Verification items for the finished model (mm, model axes). Face numbers are marked on the shaded views. A direction names the side the tool comes from. Round coordinates to 2 decimals unless told otherwise and drop trailing zeros. Order: outer loops, then holes, each group sorted by start corner. A loop starts at its lowest first (then second) coordinate and runs counter-clockwise, first axis right, second up. Notation, with made-up numbers: (-34, 68.25) -> (-30, 68.25) arc R18 ccw to (-30, 84.25) -> close; hole circle Ø4 at (-12.5, -2). An arc over 180 degrees is marked (long way). Put each result on its own line as item: value.
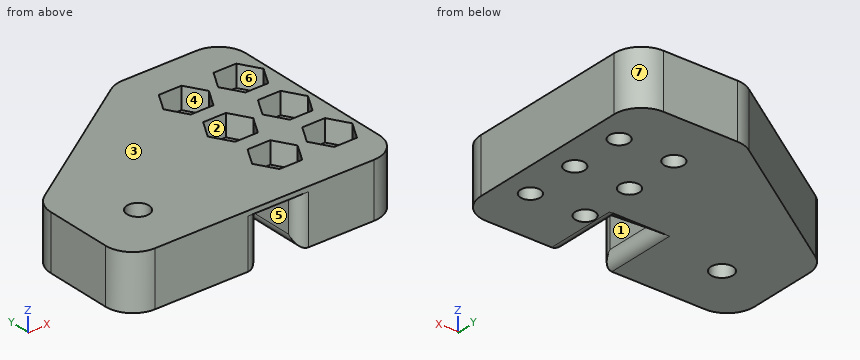
from build123d import *

# Parameters (mm, degrees)
SKETCH1_R           = 2.286
SKETCH1_R_2         = 2.54
BOSS_EXTRUDE1_DEPTH = 12.7
FILLET1_R           = 6.35
CUT_EXTRUDE1_DEPTH  = 8.89
FILLET2_R           = 2.54
CUT_EXTRUDE2_DEPTH  = 5.08


with BuildPart() as part:
    # Sketch1 → Boss-Extrude1 (new body)
    with BuildSketch(Plane.XY):
        Polygon((-6.35, 38.1), (-44.45, 12.7), (-44.45, -12.7), (-6.35, -12.7), (19.05, -12.7), (19.05, 38.1), align=None)
        Circle(SKETCH1_R, mode=Mode.SUBTRACT)
        with Locations((-31.75, 0)):
            Circle(SKETCH1_R_2, mode=Mode.SUBTRACT)
        with Locations((12.7, 0)):
            Circle(SKETCH1_R, mode=Mode.SUBTRACT)
        with Locations((12.7, 12.7)):
            Circle(SKETCH1_R, mode=Mode.SUBTRACT)
        with Locations((12.7, 25.4)):
            Circle(SKETCH1_R, mode=Mode.SUBTRACT)
        with Locations((0, 12.7)):
            Circle(SKETCH1_R, mode=Mode.SUBTRACT)
        with Locations((0, 25.4)):
            Circle(SKETCH1_R, mode=Mode.SUBTRACT)
    extrude(amount=BOSS_EXTRUDE1_DEPTH)

    # Fillet1
    fillet1_edges = [part.edges().sort_by_distance(p)[0] for p in [
        (-44.45, -12.7, 6.35),
        (-44.45, 12.7, 6.35),
        (-6.35, 38.1, 6.35),
        (19.05, 38.1, 6.35),
        (19.05, -12.7, 6.35),
    ]]
    fillet(fillet1_edges, radius=FILLET1_R)

    # Sketch2 → Cut-Extrude1 (cut)
    with BuildSketch(Plane(origin=(-5.08, 0, 0), x_dir=(0, 0, -1), z_dir=(1, 0, 0))):
        Polygon((0, 3.81), (-11.560426456, -12.7), (0, -12.7), align=None)
    extrude(amount=-CUT_EXTRUDE1_DEPTH, mode=Mode.SUBTRACT)

    # Fillet2
    fillet2_edges = [part.edges().sort_by_distance(p)[0] for p in [
        (-13.97, -4.445, 0),
        (-13.97, -12.7, 5.780213228),
        (-5.08, -4.445, 0),
        (-5.08, -12.7, 5.780213228),
    ]]
    fillet(fillet2_edges, radius=FILLET2_R)

    # Sketch3 → Cut-Extrude2 (cut)
    with BuildSketch(Plane.XY.offset(12.7)):
        Polygon((17.979290861, 0), (15.339645431, 4.572), (10.060354569, 4.572), (7.420709139, 0), (10.060354569, -4.572), (15.339645431, -4.572), align=None)
        Polygon((5.279290861, 0), (2.639645431, 4.572), (-2.639645431, 4.572), (-5.279290861, 0), (-2.639645431, -4.572), (2.639645431, -4.572), align=None)
        Polygon((17.979290861, 12.7), (15.339645431, 17.272), (10.060354569, 17.272), (7.420709139, 12.7), (10.060354569, 8.128), (15.339645431, 8.128), align=None)
        Polygon((17.979290861, 25.4), (15.339645431, 29.972), (10.060354569, 29.972), (7.420709139, 25.4), (10.060354569, 20.828), (15.339645431, 20.828), align=None)
        Polygon((5.279290861, 12.7), (2.639645431, 17.272), (-2.639645431, 17.272), (-5.279290861, 12.7), (-2.639645431, 8.128), (2.639645431, 8.128), align=None)
        Polygon((5.279290861, 25.4), (2.639645431, 29.972), (-2.639645431, 29.972), (-5.279290861, 25.4), (-2.639645431, 20.828), (2.639645431, 20.828), align=None)
    extrude(amount=-CUT_EXTRUDE2_DEPTH, mode=Mode.SUBTRACT)


solid = part.part
Item 1: Material ranges on L1, parallel to Y at x = 11, z = 9; L2, parallel to X at y = -3, z = 3.5; L3, parallel to X at y = 25.4, z = 2.25, recorded low to high. Write a range as [from, to].
Check sheet entries:
L1: y = [-12.7, -4.57], [4.57, 8.13], [17.27, 20.83], [29.97, 38.1]
L2: x = [-44.45, -13.97], [-5.08, 19.05]
L3: x = [-25.4, -2.29], [2.29, 10.41], [14.99, 19.05]
Item 2: Section check C-C on x = -24.5. Record the boundary of the cut face in (y, z).
Check sheet entries:
outline: (-12.7, 0) -> (26, 0) -> (26, 12.7) -> (-12.7, 12.7) -> close
Item 3: Section check B-B on z = 5. Record the boundary of the cut face in (x, y), then the cut area to 3 significant figures.
Check sheet entries:
outline: (-44.45, -6.35) arc R6.35 ccw to (-38.1, -12.7) -> (-16.51, -12.7) arc R2.54 ccw to (-13.97, -10.16) -> (-13.97, -3.33) -> (-5.08, -3.33) -> (-5.08, -10.16) arc R2.54 ccw to (-2.54, -12.7) -> (12.7, -12.7) arc R6.35 ccw to (19.05, -6.35) -> (19.05, 31.75) arc R6.35 ccw to (12.7, 38.1) -> (-4.43, 38.1) arc R6.35 ccw to (-7.95, 37.03) -> (-41.62, 14.59) arc R6.35 ccw to (-44.45, 9.3) -> close; hole circle Ø5.08 at (-31.75, 0); hole circle Ø4.57 at (0, 0); hole circle Ø4.57 at (0, 12.7); hole circle Ø4.57 at (0, 25.4); hole circle Ø4.57 at (12.7, 0); hole circle Ø4.57 at (12.7, 12.7); hole circle Ø4.57 at (12.7, 25.4)
area: 2,510 mm^2
Item 4: Section check A-A on x = -31.75. Record the boundary of the cut face in (y, z).
Check sheet entries:
outline: (-12.7, 0) -> (-2.54, 0) -> (-2.54, 12.7) -> (-12.7, 12.7) -> close; (2.54, 0) -> (21.17, 0) -> (21.17, 12.7) -> (2.54, 12.7) -> close
Item 5: Section check D-D on z = 8.5. State how many separate pieces and enclosed holes the cut face has, then the cut area to 3 significant figures.
Check sheet entries:
separate pieces: 1
enclosed holes: 7
area: 2,220 mm^2
Item 6: Gauge pin test, flat ends, axial feed: pin 1 Ø1.5 at (y, z) = (13.5, 11) entering from -X; pin 2 Ø10 at (x, y) = (2.5, 0) entering from +Z; pin 3 Ø3 at (y, z) = (26, 11.5) entering from -X; pin 4 Ø4 at (y, z) = (21, 2.5) entering from -X. Record the tip position at first contact, or that the pin passes through.
Check sheet entries:
pin 1: stops at x = -43.43
pin 2: stops at z = 12.7
pin 3: stops at x = -26.75
pin 4: stops at x = -35
Item 7: Tool access check on the marked faces 1, 2 and 3. Record the directions out of +Z, -Z, +X, -X, +Y, -Y that give a thin tool (end or side, any length) a straight path to the whole face; none if there is none.
Check sheet entries:
face 1: -Z, -Y
face 2: +Z
face 3: +Z, +X, -X, +Y, -Y
Item 8: Release check for a two-part mould opening along Y. For the marked faces 4, 5, 6 and 7 record: +Y half, -Y half, draft (parallel to the pull), parting line (faces both ways), or undercut.
Check sheet entries:
face 4: undercut
face 5: draft
face 6: undercut
face 7: +Y half
